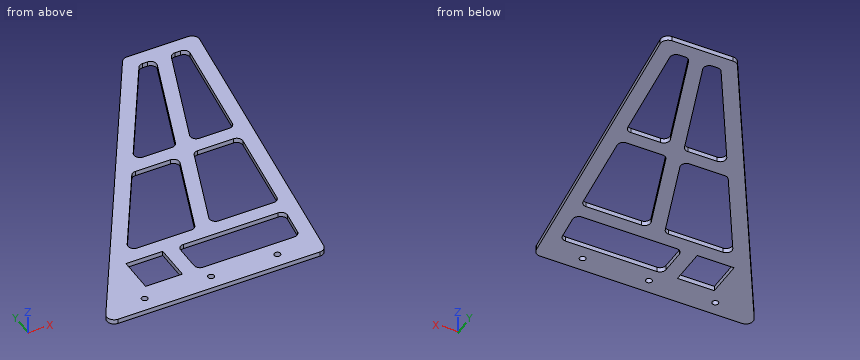
from build123d import *

# Parameters (mm, degrees)
EXTRUDE_1_DEPTH            = 3.2
FILLET_1_R                 = 5
SKETCH_2_R                 = 2.1
CUT_EXTRUDE_1_DEPTH        = 3.2
PATTERN_LINEAR_1_COUNT     = 2
PATTERN_LINEAR_1_PITCH     = 45
PATTERN_LINEAR_1_COL_COUNT = 2
PATTERN_LINEAR_1_COL_PITCH = 45
EXTRUDE_2_DEPTH            = 3.2
FILLET_2_R                 = 4


with BuildPart() as part:
    # Эскиз1 → Бобышка-Вытянуть1 (new body)
    with BuildSketch(Plane.XY):
        Polygon((0, 0), (150, 0), (180, 220), (130, 220), align=None)
        Polygon((135.706302127, 210), (23.433574854, 20), (142.634725768, 20), (168.543816677, 210), align=None, mode=Mode.SUBTRACT)
    extrude(amount=EXTRUDE_1_DEPTH)

    # Скругление1
    fillet_1_edges = [part.edges().sort_by_distance(p)[0] for p in [
        (130, 220, 1.6),
        (180, 220, 1.6),
        (150, 0, 1.6),
        (0, 0, 1.6),
    ]]
    fillet(fillet_1_edges, radius=FILLET_1_R)

    # Эскиз2 → Вырез-Вытянуть1 (cut)
    with BuildSketch(Plane.XY.offset(3.2)):
        with Locations((77.198893337, 10)):
            Circle(SKETCH_2_R)
    cut_extrude_1 = extrude(amount=-CUT_EXTRUDE_1_DEPTH, mode=Mode.SUBTRACT)

    # Линейный массив1: Вырез-Вытянуть1 ×2
    with Locations(*[(i * PATTERN_LINEAR_1_PITCH, 0, 0) for i in range(1, PATTERN_LINEAR_1_COUNT)]):
        add(cut_extrude_1, mode=Mode.SUBTRACT)

    # Линейный массив1 col: Вырез-Вытянуть1 ×2
    with Locations(*[(-i * PATTERN_LINEAR_1_COL_PITCH, 0, 0) for i in range(1, PATTERN_LINEAR_1_COL_COUNT)]):
        add(cut_extrude_1, mode=Mode.SUBTRACT)

    # Эскиз4 → Бобышка-Вытянуть2 (add)
    with BuildSketch(Plane.XY):
        Polygon((44.115393036, 55), (38.206302127, 45), (63.206302127, 45), (63.206302127, 20), (73.206302127, 20), (73.206302127, 45), (92.125059402, 45), (152.125059402, 210), (147.125059402, 210), (118.215968493, 130.5), (88.729029399, 130.5), (82.81993849, 120.5), (114.579604856, 120.5), (90.761423038, 55), align=None)
        Polygon((152.125059402, 210), (92.125059402, 45), (146.043816677, 45), (147.40745304, 55), (100.761423038, 55), (124.579604856, 120.5), (156.339271222, 120.5), (157.702907586, 130.5), (128.215968493, 130.5), (157.125059402, 210), align=None)
        Polygon((38.206302127, 45), (38.206302127, 20), (23.433574854, 20), align=None)
    extrude(amount=EXTRUDE_2_DEPTH)

    # Скругление2
    fillet_2_edges = [part.edges().sort_by_distance(p)[0] for p in [
        (147.125059402, 210, 1.6),
        (118.215968493, 130.5, 1.6),
        (88.729029399, 130.5, 1.6),
        (82.81993849, 120.5, 1.6),
        (114.579604856, 120.5, 1.6),
        (90.761423038, 55, 1.6),
        (44.115393036, 55, 1.6),
        (73.206302127, 20, 1.6),
        (168.543816677, 210, 1.6),
        (135.706302127, 210, 1.6),
        (142.634725768, 20, 1.6),
        (73.206302127, 45, 1.6),
        (146.043816677, 45, 1.6),
        (147.40745304, 55, 1.6),
        (100.761423038, 55, 1.6),
        (124.579604856, 120.5, 1.6),
        (156.339271222, 120.5, 1.6),
        (157.702907586, 130.5, 1.6),
        (128.215968493, 130.5, 1.6),
        (157.125059402, 210, 1.6),
    ]]
    fillet(fillet_2_edges, radius=FILLET_2_R)


solid = part.part
Read the model definition and answer for the solid it produces. Units are mm, in the model's axes. Give positions to 0.01 mm unless a question says otherwise; leave off trailing zeros. Loops run counter-clockwise (first coordinate to the right, second up) from the corner with the lowest first, then second, coordinate; pieces in that order, holes last. Notation, with made-up numbers: M -32,87.25 L -4,87.25 A28 ccw -4,122.25 Z; hole C 24,-37 d10. An arc over 180 degrees is marked long. Write each question's results on one line, items separated by ' | '.
1. Given pin 1 (1 mm diameter, centred on x = 64.5, z = 1, fed in from +Y); pin 2 (3.5 mm diameter, centred on x = 77.2, y = 10, fed in from -Z); pin 3 (1 mm diameter, centred on x = 107.5, z = 2, fed in from +Y); pin 4 (1 mm diameter, centred on x = 96, z = 1.5, fed in from +Y), each flat-ended and moving along its own axis, determine where each tip first touches the part or whether it passes through.
Values:
pin 1: stops at y = 110 | pin 2: passes through | pin 3: stops at y = 182.77 | pin 4: stops at y = 163.31
2. Section B-B on z = 0.65 is taken. State how many separate pieces and enclosed holes the cut face has, plus the area to 3 significant figures.
Values:
separate pieces: 1 | enclosed holes: 9 | area: 11,200 mm^2
3. Section A-A on y = 150 is taken. Give the vertices of the cut face in (x, z).
Values:
outline: M 88.64,0 L 100.25,0 L 100.25,3.2 L 88.64,3.2 Z; M 125.31,0 L 135.31,0 L 135.31,3.2 L 125.31,3.2 Z; M 160.36,0 L 170.45,0 L 170.45,3.2 L 160.36,3.2 Z
4. Straight lines are drawn through the part: line 1 (X direction, y = 119, z = 2.7); line 2 (X direction, y = 175.5, z = 1.8); line 3 (Y direction, x = 40, z = 2.7). For each, find the intervals that lie inside material, in ascending order. Write a range as [from, to].
Values:
line 1: x = [70.32, 81.98], [111.99, 124.26], [154.88, 166.23] | line 2: x = [103.7, 115.32], [134.58, 144.58], [163.84, 173.93] | line 3: y = [0, 20], [45, 67.69]
